Autodesk Inventor part; units mm, degrees
ref_plane "YZ Plane" through (0, 0, 0) normal (1, 0, 0) x (0, 1, 0)
ref_plane "XZ Plane" through (0, 0, 0) normal (0, 1, 0) x (-1, 0, 0)
ref_plane "XY Plane" through (0, 0, 0) normal (0, 0, 1) x (1, 0, 0)
sketch "Esquisse1" plane through (0, 0, 0) normal (0, 0, 1) x (1, 0, 0)
  line L0 (5.5, -5.5) -> (-5.5, -5.5) construction
  line L1 (-5.5, -5.5) -> (-5.5, 5.5) construction
  line L2 (-5.5, 5.5) -> (5.5, 5.5) construction
  line L3 (5.5, 5.5) -> (5.5, -5.5) construction
  line L4 (5.5, -5.5) -> (-5.5, 5.5) construction
  line L5 (-5.5, -5.5) -> (5.5, 5.5) construction
  circle A0 centre (-5.5, 5.5) radius 1.55
  circle A1 centre (-5.5, -5.5) radius 1.55
  circle A2 centre (5.5, 5.5) radius 1.55
  line L6 (-2.5, -8.5) -> (-8.5, -8.5)
  line L7 (-8.5, -8.5) -> (-8.5, 8.5)
  line L8 (-8.5, 8.5) -> (-2.5, 8.5)
  line L9 (-2.5, 8.5) -> (-2.5, -8.5)
  line L10 (-2.5, -8.5) -> (-8.5, 8.5) construction
  line L11 (-8.5, -8.5) -> (-2.5, 8.5) construction
  line L12 (8.5, 2.5) -> (-8.5, 2.5)
  line L13 (-8.5, 2.5) -> (-8.5, 8.5)
  line L14 (-8.5, 8.5) -> (8.5, 8.5)
  line L15 (8.5, 8.5) -> (8.5, 2.5)
  line L16 (8.5, 2.5) -> (-8.5, 8.5) construction
  line L17 (-8.5, 2.5) -> (8.5, 8.5) construction
  line L18 (-2.5, -8.5) -> (2, -8.5)
  line L19 (8.5, 2.5) -> (2, -8.5)
  point P0 (0, 0)
  point P1 (-5.5, 0)
  point P2 (0, 5.5)
  point P3 (-2.5, 8.5)
  point P4 (-2.5, 2.5)
  dimension "d0" = 11
  dimension "d1" = 3.1
  dimension "d2" = 6
  dimension "d8" = 4.5
extrude "Extrusion1" add sketch "Esquisse1" against normal blind 6 contours L6 L7 L12 L9 | L12 L7 L8 L9
extrude "Extrusion2" add sketch "Esquisse1" along normal blind 3
properties part number "Support Vis rotation"
Source: CAD feature listing. Evaluate the final solid. Frame: model axes, mm. A direction names the side the tool comes from. Coordinates: 2 decimals unless noted, no trailing zeros. Loops run counter-clockwise (first coordinate to the right, second up) from the corner with the lowest first, then second, coordinate; pieces in that order, holes last. Notation, with made-up numbers: M 83,39.25 L 128,39.25 A21 ccw 128,55.25 Z; hole C 18.5,45 d1. An arc over 180 degrees is marked long. Use CSV: the item, a comma, the result in double quotes.
(1) Cut plane B-B on y = -5.5. Return loops of the section in (x, z), and give its area (3 significant figures).
Answers follow:
outline,"M -8.5,-6 L -7.05,-6 L -7.05,3 L -8.5,3 Z; M -3.95,-6 L -2.5,-6 L -2.5,0 L 3.77,0 L 3.77,3 L -3.95,3 Z"
area,"44.9 mm²"
(2) Cut plane A-A on x = -5.5. Return loops of the section in (y, z), and give its area (3 significant figures).
Answers follow:
outline,"M -8.5,-6 L -7.05,-6 L -7.05,3 L -8.5,3 Z; M -3.95,-6 L 3.95,-6 L 3.95,3 L -3.95,3 Z; M 7.05,-6 L 8.5,-6 L 8.5,3 L 7.05,3 Z"
area,"97.2 mm²"
(3) Reachability of faces 5 (the face through (-2, 8.5, 1)), 6 (the face through (2, 0, 0)) from +Z, -Z, +X, -X, +Y, -Y: full face, straight path, thin tool, end or side. Return the list, or none.
Answers follow:
face 5,"+Z, -Z, +X, -X, +Y"
face 6,"-Z, +X, +Y, -Y"
(4) Contact query for flat-ended pins moving along their axis: pin 1 (3.5 mm diameter, centred on x = 5.5, y = 5.5, fed in from -Z); pin 2 (5 mm diameter, centred on y = -5, z = -0.5, fed in from +X); pin 3 (3 mm diameter, centred on y = 0.5, z = -2, fed in from +X); pin 4 (2.5 mm diameter, centred on x = -5.5, y = 5.5, fed in from +Z). Output: stop coordinate, or through.
Answers follow:
pin 1,"z = 0"
pin 2,"x = 5.52"
pin 3,"x = -2.5"
pin 4,"through"
(5) Draft query along X for faces 1 (the face through (-4, -8.5, 0)), 2 (the face through (5.295, -2.923, 1.479)), 3 (the face through (-8.5, 0, -1)), 4 (the face through (3.95, 5.43, 1.48)). Return one class per face: pulls with the +X half, pulls with the -X half, needs draft (parallel to the pull), parting line crosses it, or undercut.
Answers follow:
face 1,"needs draft"
face 2,"pulls with the +X half"
face 3,"pulls with the -X half"
face 4,"undercut"
(6) Cut plane C-C on z = 1. Return loops of the section in (x, y), and give its area (3 significant figures).
Answers follow:
outline,"M -8.5,-8.5 L 2,-8.5 L 8.5,2.5 L 8.5,8.5 L -8.5,8.5 Z; hole C -5.5,-5.5 d3.1; hole C -5.5,5.5 d3.1; hole C 5.5,5.5 d3.1"
area,"231 mm²"
(7) Line query: line 1 (Y direction, x = -5.5, z = 0.75); line 2 (Z direction, x = -1.5, y = 5.25); line 3 (Y direction, x = -6.5, z = 1). Output: solid intervals per line, ascending. Write a range as [from, to].
Answers follow:
line 1,"[-8.5, -7.05], [-3.95, 3.95], [7.05, 8.5]"
line 2,"[0, 3]"
line 3,"[-8.5, -6.68], [-4.32, 4.32], [6.68, 8.5]"
(8) Cut plane D-D on z = -3.75. Return loops of the section in (x, y), and give its area (3 significant figures).
Answers follow:
outline,"M -8.5,-8.5 L -2.5,-8.5 L -2.5,8.5 L -8.5,8.5 Z; hole C -5.5,-5.5 d3.1; hole C -5.5,5.5 d3.1"
area,"86.9 mm²"
